Can you work these out from the model? Positions are in its coordinate system, mm. Give positions to 0.01 mm unless a question says otherwise; leave off trailing zeros. Order: outer loops, then holes, each group sorted by start corner. A loop starts at its lowest first (then second) coordinate and runs counter-clockwise, first axis right, second up.
Item 1: If I drill on line 1 along Y through (x, z) = (0, 1.4); line 2 along X through (y, z) = (10, 3); line 3 along X through (y, z) = (24.5, 0.3), over which ranges is the centre line in solid material (lowest first)?
Item 2: I want a section at B-B, the plane y = -25.4. Write out the boundary of the cut face in (x, z) (3 decimals), then the cut area to 3 significant figures.
Item 3: I want a section at A-A, the plane x = 0. Write out the boundary of the cut face in (y, z) (1 decimal), then the cut area to 3 significant figures.
Item 4: I want a section at D-D, the plane y = 88.9. Write out the boundary of the cut face in (x, z) (1 decimal), then the cut area to 3 significant figures.
Item 5: I'm going to push flat-ended pins straight in: pin 1 Ø4 at (x, y) = (2.5, 17.5) entering from -Z; pin 2 Ø1.6 at (y, z) = (0, 2) entering from +X. Where does each tip first touch, or does it pass through?
Item 6: I want a section at C-C, the plane z = 1.2. Write out the boundary of the cut face in (x, y) (1 decimal).
Item 7: If we mould it in two halves opening along Y, with no side actions, what happens to faces 1 (the cylindrical face through (-3.097, 74.952, 1.61)), 2 (the flat face through (50.71, 81.12, 1.57)), 3 (the flat face through (25, 82, 3.175))? For each: +Y half, -Y half, draft (parallel to the pull), parting line (faces both ways), or undercut.
```python
from build123d import *

# Parameters (mm, degrees)
BOSS_EXTRUDE1_DEPTH = 3.175
SKETCH2_R           = 3.3734375
CUT_EXTRUDE1_DEPTH  = 3.175
SKETCH3_R           = 2.4638
CUT_EXTRUDE2_DEPTH  = 3.175
SKETCH4_R           = 14.2875
CUT_EXTRUDE3_DEPTH  = 3.175
CUT_EXTRUDE4_DEPTH  = 222.091497051
FILLET1_R           = 2.54


with BuildPart() as part:
    # Sketch1 → Boss-Extrude1 (new body)
    with BuildSketch(Plane.XY):
        Polygon((49.741526937, 199.241524535), (10.132643551, 114.3), (-25.4, 114.3), (-25.4, 38.1), (-25.4, -38.1), (25.4, -38.1), (25.4, 26.837911138), (95.781962519, 177.772516839), align=None)
    extrude(amount=BOSS_EXTRUDE1_DEPTH)

    # Sketch2 → Cut-Extrude1 (cut)
    with BuildSketch(Plane.XY.offset(3.175)):
        with Locations((62.02724088, 165.486802896)):
            Circle(SKETCH2_R)
    extrude(amount=-CUT_EXTRUDE1_DEPTH, mode=Mode.SUBTRACT)

    # Sketch3 → Cut-Extrude2 (cut)
    with BuildSketch(Plane.XY.offset(3.175)):
        with Locations((0, -25.4)):
            Circle(SKETCH3_R)
        Circle(SKETCH3_R)
        with Locations((0, 25.4)):
            Circle(SKETCH3_R)
    extrude(amount=-CUT_EXTRUDE2_DEPTH, mode=Mode.SUBTRACT)

    # Sketch4 → Cut-Extrude3 (cut)
    with BuildSketch(Plane.XY.offset(3.175)):
        with Locations((0, 88.9)):
            Circle(SKETCH4_R)
    extrude(amount=-CUT_EXTRUDE3_DEPTH, mode=Mode.SUBTRACT)

    # Sketch5 → Cut-Extrude4 (cut, through all)
    with BuildSketch(Plane.XY.offset(3.175)):
        Polygon((76.731962519, 186.655677727), (76.731962519, 136.919660003), (95.781962519, 177.772516839), align=None)
    extrude(amount=-CUT_EXTRUDE4_DEPTH, mode=Mode.SUBTRACT)

    # Fillet1
    fillet1_edges = [part.edges().sort_by_distance(p)[0] for p in [
        (10.132643551, 114.3, 1.5875),
        (49.741526937, 199.241524535, 1.5875),
        (25.4, 26.837911138, 1.5875),
        (25.4, -38.1, 1.5875),
        (-25.4, -38.1, 1.5875),
        (-25.4, 114.3, 1.5875),
        (76.731962519, 186.655677727, 1.5875),
        (76.731962519, 136.919660003, 1.5875),
    ]]
    fillet(fillet1_edges, radius=FILLET1_R)


solid = part.part
```
Results list:
1. line 1: y = -38.1 to -27.86, -22.94 to -2.46, 2.46 to 22.94, 27.86 to 74.61, 103.19 to 114.3
1. line 2: x = -25.4 to 25.4
1. line 3: x = -25.4 to -2.29, 2.29 to 25.4
2. outline: (-25.4, 0) - (-2.464, 0) - (-2.464, 3.175) - (-25.4, 3.175) - close; (2.464, 0) - (25.4, 0) - (25.4, 3.175) - (2.464, 3.175) - close
2. area: 146 mm2
3. outline: (-38.1, 0) - (-27.9, 0) - (-27.9, 3.2) - (-38.1, 3.2) - close; (-22.9, 0) - (-2.5, 0) - (-2.5, 3.2) - (-22.9, 3.2) - close; (2.5, 0) - (22.9, 0) - (22.9, 3.2) - (2.5, 3.2) - close; (27.9, 0) - (74.6, 0) - (74.6, 3.2) - (27.9, 3.2) - close; (103.2, 0) - (114.3, 0) - (114.3, 3.2) - (103.2, 3.2) - close
3. area: 346 mm2
4. outline: (-25.4, 0) - (-14.3, 0) - (-14.3, 3.2) - (-25.4, 3.2) - close; (14.3, 0) - (54.3, 0) - (54.3, 3.2) - (14.3, 3.2) - close
4. area: 162 mm2
5. pin 1: stops at z = 0
5. pin 2: stops at x = 25.4
6. outline: (-25.4, -35.6) arc R2.5 ccw to (-22.9, -38.1) - (22.9, -38.1) arc R2.5 ccw to (25.4, -35.6) - (25.4, 26.3) arc R2.5 cw to (25.6, 27.3) - (76.5, 136.4) arc R2.5 ccw to (76.7, 137.5) - (76.7, 185) arc R2.5 ccw to (75.3, 187.3) - (52, 198.2) arc R2.5 ccw to (48.7, 196.9) - (10.8, 115.8) arc R2.5 cw to (8.5, 114.3) - (-22.9, 114.3) arc R2.5 ccw to (-25.4, 111.8) - close; hole circle Ø28.6 at (0, 88.9); hole circle Ø4.9 at (0, -25.4); hole circle Ø4.9 at (0, 0); hole circle Ø4.9 at (0, 25.4); hole circle Ø6.7 at (62, 165.5)
7. face 1: undercut
7. face 2: -Y half
7. face 3: draft
